Part print with two shaded views. Sizes in mm from the minimum x, y, z corner. A direction names the side the tool comes from. Coordinates: 2 decimals unless noted, no trailing zeros. Order: outer loops, then holes, each group sorted by start corner. A loop starts at its lowest first (then second) coordinate and runs counter-clockwise, first axis right, second up. Notation, with made-up numbers: (70, 15) - (80, 15) arc R13 cw to (80, 19) - close; hole circle Ø5 at (35, -10.5). An arc over 180 degrees is marked (long way). One line per item, written item: value.
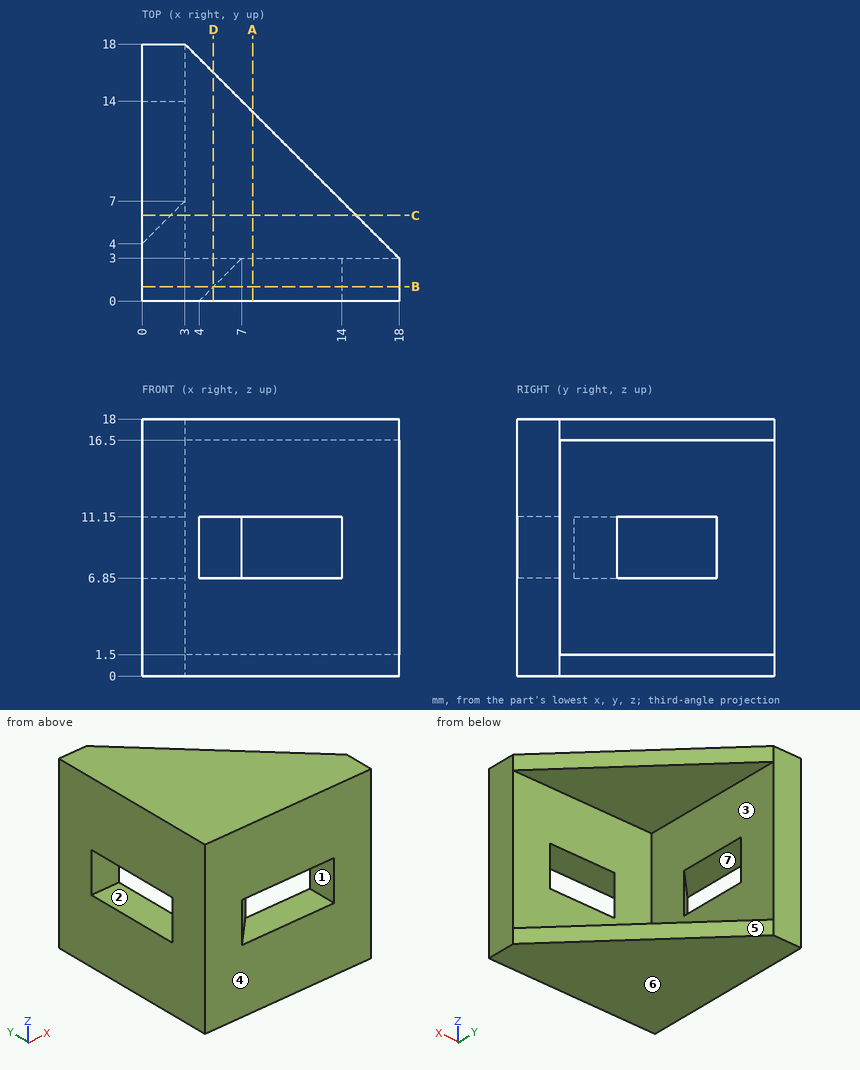
1. 3-axis set-ups, long thin cutter, end or side, ignore diameter. For the marked faces 1, 2 and 3: which of +Z, -Z, +X, -X, +Y, -Y reach the whole face in a straight line?
Values found:
face 1: +Y, -Y
face 2: -X
face 3: +X, +Y
2. Band-saw the part on C-C, the plane y = 6. Give the cut face in (x, z).
Values found:
outline: (0, 0) - (15, 0) - (15, 1.5) - (3, 1.5) - (3, 16.5) - (15, 16.5) - (15, 18) - (0, 18) - (0, 11.15) - (2, 11.15) - (2, 6.85) - (0, 6.85) - close
3. Band-saw the part on B-B, the plane y = 1. Give the cut face in (x, z).
Values found:
outline: (0, 0) - (18, 0) - (18, 18) - (0, 18) - close; hole (5, 6.85) - (14, 6.85) - (14, 11.15) - (5, 11.15) - close
4. Two-plate mould, pull along Y, no slides. Class the marked faces 4, 5, 6 and 7: pulls with the +Y half, pulls with the -Y half, needs draft (parallel to the pull), parting line crosses it, or undercut.
Values found:
face 4: pulls with the -Y half
face 5: pulls with the +Y half
face 6: needs draft
face 7: undercut
5. Band-saw the part on A-A, the plane x = 7.75. Give the cut face in (y, z).
Values found:
outline: (0, 0) - (13.25, 0) - (13.25, 1.5) - (3, 1.5) - (3, 6.85) - (0, 6.85) - close; (0, 11.15) - (3, 11.15) - (3, 16.5) - (13.25, 16.5) - (13.25, 18) - (0, 18) - close
6. Band-saw the part on D-D, the plane x = 5. Give the cut face in (y, z).
Values found:
outline: (0, 0) - (16, 0) - (16, 1.5) - (3, 1.5) - (3, 16.5) - (16, 16.5) - (16, 18) - (0, 18) - (0, 11.15) - (1, 11.15) - (1, 6.85) - (0, 6.85) - close
7. Probe line 1 along Z through (x, y) = (11, 3.25); line 2 along Z through (x, y) = (1.5, 12.25); line 3 along X through (y, z) = (6.5, 6.25). List the from-to ranges inside material, lowest first.
Values found:
line 1: z = 0 to 1.5, 16.5 to 18
line 2: z = 0 to 6.85, 11.15 to 18
line 3: x = 0 to 3
8. Flat gauge pins, fed straight in: P1, Ø2, axis at y = 16, z = 16, coming from the +X side; P2, Ø1, axis at x = 10.5, z = 5.5, coming from the +Y side. Where does each tip first touch, or does it go through?
Values found:
P1: stops at x = 5.87
P2: stops at y = 3
